Read the model definition and answer for the solid it produces. Units are mm, in the model's axes. A direction names the side the tool comes from. Coordinates: 2 decimals unless noted, no trailing zeros. Loops run counter-clockwise (first coordinate to the right, second up) from the corner with the lowest first, then second, coordinate; pieces in that order, holes last.
Q1. Section D-D (y = -125) is taken. Give the vertices of the cut face in (x, z).
Q2. Which of the six approach directions +Z, -Z, +X, -X, +Y, -Y give full straight-line access (tool end or side, diameter ignored) to faces 4 (the face through (195.148, -157.287, 84.484)), 5 (the face through (198, 80, 43)), 6 (the face through (173, 79, 43)), 7 (the face through (188, 29.706, 43)), 8 (the face through (-25, -140.294, 43))?
Q3. Section B-B (z = 63.5) is taken. Give the vertices of the cut face in (x, y), then the cut area to 3 significant figures.
Q4. Straight lines are drawn through the part: line 1 (X direction, y = 76, z = 77.5); line 2 (Y direction, x = -26.5, z = 15); line 3 (X direction, y = -14, z = 12). For each, find the intervals that lie inside material, in ascending order.
Q5. Flat-ended cylindrical pins translate along their axes: P1, Ø10, axis at y = -37.5, z = 51, coming from the -X side; P2, Ø6, axis at x = 46, z = 46, coming from the -Y side; P3, Ø8, axis at x = 51, z = 77.5, coming from the +Y side. Find the tip coordinate at first contact, or state that the pin passes through.
Q6. Section C-C (x = -3) is taken. Give the vertices of the cut face in (y, z).
Q7. The mould has two halves that part along X. Classify faces 1 (the face through (183, -106.294, 43)), 2 (the face through (195.148, -157.287, 2.465)), 3 (the face through (40, -153, 5)): pulls with the +X half, pulls with the -X half, needs draft (parallel to the pull), parting line crosses it, or undercut.
Q8. Section A-A (y = -38.5) is taken. Give the vertices of the cut face in (x, z), then the cut area to 3 significant figures.
from build123d import *

# Parameters (mm, degrees)
SKETCH1_W           = 20
SKETCH1_H           = 72
BOSS_EXTRUDE2_DEPTH = 87
SKETCH2_W           = 77.037941343
SKETCH2_H           = 18.412852551
CUT_EXTRUDE1_DEPTH  = 420


with BuildPart() as part:
    # Sketch1 → Boss-Extrude2 (new body)
    with BuildSketch(Plane.XY):
        with BuildLine():
            Line((-202, -150.294090379), (-202, -140.294090379))
            Line((-202, -140.294090379), (148, -140.294090379))
            Line((148, -140.294090379), (158, -140.294090379))
            ThreePointArc((158, -140.294090379), (165.071067812, -137.36515819), (168, -130.294090379))
            Line((168, -130.294090379), (168, 129.705909621))
            Line((168, 129.705909621), (198, 129.705909621))
            Line((198, 129.705909621), (198, 29.705909621))
            Line((198, 29.705909621), (178, 29.705909621))
            Line((178, 29.705909621), (178, -20.294090379))
            Line((178, -20.294090379), (198, -20.294090379))
            Line((198, -20.294090379), (198, -150.294090379))
            ThreePointArc((198, -150.294090379), (195.071067812, -157.36515819), (188, -160.294090379))
            Line((188, -160.294090379), (-12, -160.294090379))
            Line((-12, -160.294090379), (-202, -150.294090379))
        make_face()
        with Locations((183, -70.294090379)):
            Rectangle(SKETCH1_W, SKETCH1_H, mode=Mode.SUBTRACT)
        with Locations((183, 79.705909621)):
            Rectangle(SKETCH1_W, SKETCH1_H, mode=Mode.SUBTRACT)
    extrude(amount=BOSS_EXTRUDE2_DEPTH)

    # Sketch2 → Cut-Extrude1 (cut)
    with BuildSketch(Plane.ZY.offset(202)):
        with Locations((43.518970671, -154.500516655)):
            Rectangle(SKETCH2_W, SKETCH2_H)
    extrude(amount=-CUT_EXTRUDE1_DEPTH, mode=Mode.SUBTRACT)


solid = part.part
Numbers:
1. outline: (168, 0) - (198, 0) - (198, 87) - (168, 87) - close
2. face 4: +Z, -Z, +X, -Y
2. face 5: +Z, -Z, +X, +Y, -Y
2. face 6: +Z, -Z
2. face 7: +Z, -Z, +X
2. face 8: +Z, -Z, -X, +Y
3. outline: (-202, -145.29) - (198, -145.29) - (198, -20.29) - (178, -20.29) - (178, 29.71) - (198, 29.71) - (198, 129.71) - (168, 129.71) - (168, -130.29) arc R10 cw to (158, -140.29) - (-202, -140.29) - close; hole (173, -106.29) - (193, -106.29) - (193, -34.29) - (173, -34.29) - close; hole (173, 43.71) - (193, 43.71) - (193, 115.71) - (173, 115.71) - close
3. area: 6,240 mm2
4. line 1: x = 168 to 173, 193 to 198
4. line 2: y = -145.29 to -140.29
4. line 3: x = 168 to 178
5. P1: stops at x = 168
5. P2: stops at y = -145.29
5. P3: stops at y = -140.29
6. outline: (-160.29, 0) - (-140.29, 0) - (-140.29, 87) - (-160.29, 87) - (-160.29, 82.04) - (-145.29, 82.04) - (-145.29, 5) - (-160.29, 5) - close
7. face 1: undercut
7. face 2: pulls with the +X half
7. face 3: needs draft
8. outline: (168, 0) - (173, 0) - (173, 87) - (168, 87) - close; (193, 0) - (198, 0) - (198, 87) - (193, 87) - close
8. area: 870 mm2
